Autodesk Inventor part; units mm, degrees
ref_plane "YZ Plane" through (0, 0, 0) normal (1, 0, 0) x (0, 1, 0)
ref_plane "XZ Plane" through (0, 0, 0) normal (0, 1, 0) x (-1, 0, 0)
ref_plane "XY Plane" through (0, 0, 0) normal (0, 0, 1) x (1, 0, 0)
sketch "Sketch1" plane through (0, 0, 0) normal (0, 0, 1) x (1, 0, 0)
  line L0 (254, 0) -> (254, 20)
  line L1 (254, 20) -> (0, 20)
  line L2 (0, 20) -> (0, 0)
  line L3 (0, 20) -> (0, 16) construction
  line L4 (0, 16) -> (8.5, 16) construction
  line L5 (8.5, 16) -> (11.75, 16) construction
  line L6 (11.75, 16) -> (11.75, 12.75) construction
  circle A0 centre (11.75, 12.75) radius 3.25
  line L7 (254, 20) -> (254, 16) construction
  line L8 (254, 16) -> (245.5, 16) construction
  line L9 (245.5, 16) -> (245.5, 12.75) construction
  line L10 (245.5, 12.75) -> (242.25, 12.75) construction
  circle A1 centre (242.25, 12.75) radius 3.25
  line L11 (0, 0) -> (254, 0)
  line L12 (127, 0) -> (127, -50) construction
  line L13 (122, -50) -> (132, -50)
  line L14 (132, -50) -> (132, -59)
  line L15 (122, -50) -> (122, -59)
  line L16 (132, -59) -> (136, -59)
  line L17 (122, -59) -> (118, -59)
  line L18 (118, -59) -> (118, 0)
  line L19 (136, -59) -> (136, 0)
  dimension "d1" = 20
  dimension "d2" = 4
  dimension "d3" = 8.5
  dimension "d4" = 3.25
  dimension "d5" = 3.25
  dimension "d6" = 4
  dimension "d7" = 8.5
  dimension "d8" = 3.25
  dimension "d9" = 3.25
  dimension "d14" = 242.25
  dimension "d40" = 50
  dimension "d41" = 10
  dimension "d42" = 5
  dimension "d43" = 0
  dimension "d44" = 9
  dimension "d45" = 9
  dimension "d46" = 4
  dimension "d47" = 4
extrude "Extrusion1" add sketch "Sketch1" along normal blind 8
fillet "Fillet2" radius 4 4 edges at (120, -59, 8) (120, -59, 0) (134, -59, 0) (134, -59, 8)
hole "Hole1" at (136, -55, 4) direction (-1, 0, 0) diameter 3 end through all
fillet "Fillet5" radius 10 4 edges at (0, 0, 4) (118, 0, 4) (136, 0, 4) (254, 0, 4)
fillet "Fillet6" radius 3 2 edges at (127, -50, 8) (127, -50, 0)
equation "\"d42\" = 0.5 * d41"
equation "\"d45\" = d44"
equation "\"d47\" = d46"
properties part number "WebcamBase"
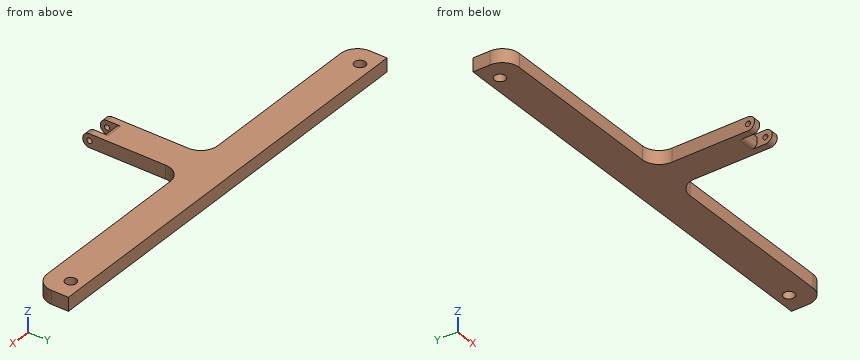
Model file for the job. Use its own axes, mm. Round coordinates to 2 decimals unless told otherwise and drop trailing zeros. Write each loop counter-clockwise with the first axis right and the second up, starting at its lowest first coordinate (ties: lowest second). Pieces come first, ordered by that corner, then holes. Notation, with made-up numbers: (-35, 61.5) - (-21, 61.5) arc R17 cw to (-21, 65.5) - close; hole circle Ø6 at (76.25, 1.25). An arc over 180 degrees is marked (long way). One line per item, written item: value.
(1) Cut at C-C, the plane y = -22. Give the cut face in (x, z), plus the area to 3 significant figures.
Values follow:
outline: (118, 0) - (136, 0) - (136, 8) - (118, 8) - close
area: 144 mm²
(2) Drop flat-ended pins along their axis: P1, Ø4, axis at y = -39, z = 3, coming from the -X side; P2, Ø8.5, axis at x = 11.75, y = 12.75, coming from the -Z side; P3, Ø5, axis at x = 242.25, y = 12.75, coming from the +Z side; P4, Ø3, axis at y = -25, z = 2.5, coming from the +X side. Give the stop position or say it passes through.
Values follow:
P1: stops at x = 118
P2: stops at z = 0
P3: passes through
P4: stops at x = 136
(3) Cut at B-B, the plane x = 21. Give the cut face in (y, z), plus the area to 3 significant figures.
Values follow:
outline: (0, 0) - (20, 0) - (20, 8) - (0, 8) - close
area: 160 mm²
(4) Wall check: probe 1 along Y at (x, z) = (121, 4); probe 2 along X at (y, z) = (12.5, 4); probe 3 along Y at (x, z) = (11.75, 2). Give the ranges that are in metal, low to high.
Values follow:
probe 1: y = -59 to -56.5, -53.5 to 20
probe 2: x = 0 to 8.51, 14.99 to 239.01, 245.49 to 254
probe 3: y = 0 to 9.5, 16 to 20
(5) Cut at A-A, the plane y = 12.75. Give the cut face in (x, z), plus the area to 3 significant figures.
Values follow:
outline: (0, 0) - (8.5, 0) - (8.5, 8) - (0, 8) - close; (15, 0) - (239, 0) - (239, 8) - (15, 8) - close; (245.5, 0) - (254, 0) - (254, 8) - (245.5, 8) - close
area: 1,930 mm²
